Input: part model. Units: mm. Frame: model coordinates. Face numbers are marked on the shaded views. A direction names the side the tool comes from. Give positions to 0.01 mm unless a question says otherwise; leave off trailing zeros. Loops run counter-clockwise (first coordinate to the right, second up) from the corner with the lowest first, then second, coordinate; pieces in that order, holes last. Notation, with made-up numbers: (-14, 59.25) -> (40, 59.25) arc R20 ccw to (40, 72.25) -> close; hole circle Ø1 at (56.5, 43.25). An arc over 180 degrees is marked (long way). Answer as a JSON object with one key per item and string values.
```python
from build123d import *

# Parameters (mm, degrees)
BOSS_EXTRUDE1_START = 3.175
SKETCH3_R           = 5.55625
SKETCH3_R_2         = 2.4003
BOSS_EXTRUDE1_DEPTH = 1.5875
BOSS_EXTRUDE2_START = 1.5875
SKETCH4_R           = 3.9751
SKETCH4_R_2         = 2.4003
BOSS_EXTRUDE2_DEPTH = 4.7625
CHAMFER1_SIZE       = 0.072009


with BuildPart() as part:
    # Sketch3 → Boss-Extrude1 (new body)
    with BuildSketch(Plane.XY.offset(BOSS_EXTRUDE1_START)):
        Circle(SKETCH3_R)
        Circle(SKETCH3_R_2, mode=Mode.SUBTRACT)
    extrude(amount=-BOSS_EXTRUDE1_DEPTH)

    # Sketch4 → Boss-Extrude2 (add)
    with BuildSketch(Plane.XY.offset(BOSS_EXTRUDE2_START)):
        Circle(SKETCH4_R)
        Circle(SKETCH4_R_2, mode=Mode.SUBTRACT)
    extrude(amount=-BOSS_EXTRUDE2_DEPTH)

    # Chamfer1
    chamfer1_edges = [part.edges().sort_by_distance(p)[0] for p in [
        (-2.4003, 0, -3.175),
        (-3.9751, 0, 1.5875),
        (-5.55625, 0, 3.175),
        (-5.55625, 0, 1.5875),
        (-2.4003, 0, 3.175),
        (-3.9751, 0, -3.175),
    ]]
    chamfer(chamfer1_edges, length=CHAMFER1_SIZE)


solid = part.part
```
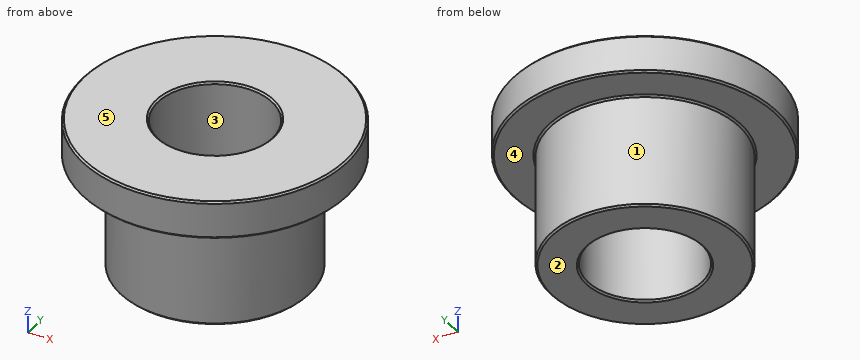
Q1. Section D-D, the plane z = -2. Return the cut outline in (x, y).
Evaluation:
{"outline": "circle Ø7.95 at (0, 0); hole circle Ø4.8 at (0, 0)"}
Q2. Section C-C, the plane z = 2. Return the cut outline in (x, y).
Evaluation:
{"outline": "circle Ø11.11 at (0, 0); hole circle Ø4.8 at (0, 0)"}
Q3. Access query for the marked faces 4 and 5. Directions: +Z, -Z, +X, -X, +Y, -Y. A direction counts if a zero-diameter tool reaches every point of the face in a straight line with its end or side. Return the directions, or none.
Evaluation:
{"face 4": "-Z", "face 5": "+Z, +X, -X, +Y, -Y"}
Q4. Pin query (flat end, axial travel): pin 1 (1.5 mm diameter, centred on x = -1.5, z = 1.5, fed in from -Y); pin 2 (1 mm diameter, centred on y = 0.5, z = -1, fed in from -X). Return the tip coordinate at first contact, or that it passes through.
Evaluation:
{"pin 1": "stops at y = -5.5", "pin 2": "stops at x = -3.98"}
Q5. Draft query along X for the marked faces 1, 2 and 3. Return one class per face: +X half, -X half, draft (parallel to the pull), parting line (faces both ways), or undercut.
Evaluation:
{"face 1": "parting line", "face 2": "draft", "face 3": "undercut"}
Q6. Ray query, line 1 along Y through (x, z) = (0, -0.25); line 2 along Z through (x, y) = (3.5, -3.5) (1 decimal); line 3 along X through (y, z) = (-0.25, -1). Return the intervals inside material, ascending.
Evaluation:
{"line 1": "y = -3.98 to -2.4, 2.4 to 3.98", "line 2": "z = 1.6 to 3.2", "line 3": "x = -3.97 to -2.39, 2.39 to 3.97"}
